CAD build for the part. Positions are in the model's coordinates, mm. A direction names the side the tool comes from. Round coordinates to 2 decimals unless told otherwise and drop trailing zeros. Write each loop counter-clockwise with the first axis right and the second up, starting at its lowest first coordinate (ties: lowest second). Pieces come first, ordered by that corner, then holes. Notation, with made-up numbers: (23, 38) - (35, 38) arc R27 cw to (35, 58) - close; hole circle Ø8 at (-12.5, 4). An arc over 180 degrees is marked (long way). Put each result on its own line as item: value. Start each with the question number.
Item 1: Pin check, flat tips, straight feed: pin 1 Ø2 at (x, y) = (6.5, -2) entering from -Z; pin 2 Ø3 at (x, y) = (4, -0.5) entering from -Z. Stop position of each tip, or through.
Item 2: 3-axis set-ups, long thin cutter, end or side, ignore diameter. For faces 1 (the cylindrical face through (8.075, -0.195, 1.487)), 2 (the flat face through (14, 0, 0)), 3 (the flat face through (1, 1, 0)): which of +Z, -Z, +X, -X, +Y, -Y reach the whole face in a straight line?
Item 3: Cut at A-A (x = 13). Give the cut face in (y, z), and give its area (3 significant figures).
Item 4: Mould opens along Z. For faces 4 (the cylindrical face through (0.203, -0.596, -2.685)), 5 (the flat face through (1, 0, -1)), 6 (the flat face through (0, -1, -1)) say: released by +Z, released by -Z, zero draft, split by the parting line, or undercut.
Item 5: Drill centre lines: line 1 (Z direction, x = 3, y = 0.45); line 2 (Y direction, x = 10.5, z = 0.9); line 3 (Y direction, x = 10.5, z = 1.35). Where is each one in solid material? Low to high. Write a range as from..to.
```python
from build123d import *

# Parameters (mm, degrees)
FILLET1_R    = 0.8
SKETCH3_W    = 0.74
SKETCH3_H    = 3
SKETCH4_W    = 0.74
SKETCH4_H    = 0.99570227
RECPAT_COUNT = 2
RECPAT_ANGLE = 90


with BuildPart() as part:
    # BodySke → Base-Revolve (revolve)
    with BuildSketch(Plane.XY):
        Polygon((0, 0), (0, 2.75), (0.4, 2.75), (1.65, 1.5), (14, 1.5), (14, 0), align=None)
    revolve(axis=Axis((-6.35, 0, 0), (1, 0, 0)))

    # Fillet1
    fillet1_edges = [part.edges().sort_by_distance(p)[0] for p in [
        (1.65, -1.5, 0),
    ]]
    fillet(fillet1_edges, radius=FILLET1_R)

    # Sketch3 → Recess section 0
    with BuildSketch(Plane.ZY):
        Rectangle(SKETCH3_W, SKETCH3_H)
    # Sketch4 → Recess section 1
    with BuildSketch(Plane.ZY.offset(-2.01)):
        Rectangle(SKETCH4_W, SKETCH4_H)
    recess = loft(mode=Mode.SUBTRACT)

    # RecPat: Recess ×2 about axis
    recpat_axis = Axis((0, 0, 0), (1, 0, 0))
    for i in range(1, RECPAT_COUNT):
        add(recess.rotate(recpat_axis, i * RECPAT_ANGLE / (RECPAT_COUNT - 1)), mode=Mode.SUBTRACT)

    # RecCorSke → RecessCore (revolve, cut)
    with BuildSketch(Plane.XY):
        Polygon((0, 0), (0, 0.696552892), (2.01, 0.556), (2.190655351, 0), align=None)
    revolve(axis=Axis((-3.175, 0, 0), (1, 0, 0)), mode=Mode.SUBTRACT)


solid = part.part
```
Output values:
1. pin 1: z = -1.12
1. pin 2: z = -1.5
2. face 1: +X
2. face 2: +Z, -Z, +X, +Y, -Y
2. face 3: -X
3. outline: circle Ø3 at (0, 0)
3. area: 7.07 mm2
4. face 4: split by the parting line
4. face 5: undercut
4. face 6: zero draft
5. line 1: -1.43..1.43
5. line 2: -1.2..1.2
5. line 3: -0.65..0.65
